from build123d import *

# Parameters (mm, degrees)
ESQUISSE1_W             = 200
ESQUISSE1_H             = 150
BOSS_EXTRU_1_DEPTH      = 1.6
ESQUISSE2_R             = 2.5
ESQUISSE2_R_2           = 2.6
ENL_V_MAT_EXTRU_1_DEPTH = 10


with BuildPart() as part:
    # Esquisse1 → Boss.-Extru.1 (new body)
    with BuildSketch(Plane.XY):
        Rectangle(ESQUISSE1_W, ESQUISSE1_H)
    extrude(amount=BOSS_EXTRU_1_DEPTH)

    # Esquisse2 → Enlèv. mat.-Extru.1 (cut)
    with BuildSketch(Plane(origin=(0, 0, 0), x_dir=(-1, 0, 0), z_dir=(0, 0, -1))):
        with Locations((75.3, -0.196647834)):
            Circle(ESQUISSE2_R)
        with Locations((25.3, -0.196647834)):
            Circle(ESQUISSE2_R)
        with Locations((-24.7, -0.196647834)):
            Circle(ESQUISSE2_R_2)
        with Locations((-74.7, -0.196647834)):
            Circle(ESQUISSE2_R)
        with Locations((75.3, -68.196647834)):
            Circle(ESQUISSE2_R)
        with Locations((25.3, -68.196647834)):
            Circle(ESQUISSE2_R)
        with Locations((-24.7, -68.196647834)):
            Circle(ESQUISSE2_R)
        with Locations((-74.7, -68.196647834)):
            Circle(ESQUISSE2_R)
    extrude(amount=-ENL_V_MAT_EXTRU_1_DEPTH, mode=Mode.SUBTRACT)


solid = part.part
For this review, take the finished solid that the model builds, in its own axes (mm). Round coordinates to 2 decimals unless told otherwise and drop trailing zeros. Write each loop counter-clockwise with the first axis right and the second up, starting at its lowest first coordinate (ties: lowest second). Pieces come first, ordered by that corner, then holes. Notation, with made-up numbers: (22, -2) -> (32, -2) arc R16 ccw to (32, 7) -> close; hole circle Ø8 at (14, -11). An arc over 180 degrees is marked (long way). Put each result on its own line as item: value.
Q1. To check wall thickness, follow L1, parallel to Y at x = 74.7, z = 1. State the ranges of the line that lie inside material, in increasing order. Write a range as [from, to].
Determined:
L1: y = [-75, -70.7], [-65.7, -2.7], [2.3, 75]
Q2. Consider section A-A on x = 24.7. State the section outline as (y, z) points.
Determined:
outline: (-75, 0) -> (-70.7, 0) -> (-70.7, 1.6) -> (-75, 1.6) -> close; (-65.7, 0) -> (-2.8, 0) -> (-2.8, 1.6) -> (-65.7, 1.6) -> close; (2.4, 0) -> (75, 0) -> (75, 1.6) -> (2.4, 1.6) -> close
Q3. Consider section B-B on x = 74.7. State the section outline as (y, z) points, and give its area (3 significant figures).
Determined:
outline: (-75, 0) -> (-70.7, 0) -> (-70.7, 1.6) -> (-75, 1.6) -> close; (-65.7, 0) -> (-2.7, 0) -> (-2.7, 1.6) -> (-65.7, 1.6) -> close; (2.3, 0) -> (75, 0) -> (75, 1.6) -> (2.3, 1.6) -> close
area: 224 mm^2
Q4. The part is to be moulded in two halves that separate along X. For faces 1 (the flat face through (-1, 1, 1.6)), 2 (the cylindrical face through (25.242, -70.637, 0.789)), say which applies: released by +X, released by -X, zero draft, split by the parting line, or undercut.
Determined:
face 1: zero draft
face 2: undercut
